Verification items for the finished model (mm, model axes). A direction names the side the tool comes from. Give positions to 0.01 mm unless a question says otherwise; leave off trailing zeros. Write each loop counter-clockwise with the first axis right and the second up, starting at its lowest first coordinate (ties: lowest second). Pieces come first, ordered by that corner, then holes. Notation, with made-up numbers: (-1, -10) -> (14, -10) arc R24 cw to (14, 0) -> close; hole circle Ø4 at (17, -29). An arc over 180 degrees is marked (long way). Use CSV: the item, a comma, the result in double quotes. Start each with the question number.
```python
from build123d import *

# Parameters (mm, degrees)
SKETCH1_W           = 17.5
SKETCH1_H           = 7.5
BOSS_EXTRUDE1_DEPTH = 8.5
SKETCH2_W           = 5.5
SKETCH2_H           = 3.8
BOSS_EXTRUDE2_DEPTH = 5
FILLET1_R           = 1
FILLET2_R           = 1


with BuildPart() as part:
    # Sketch1 → Boss-Extrude1 (new body)
    with BuildSketch(Plane.XY):
        Rectangle(SKETCH1_W, SKETCH1_H)
    extrude(amount=BOSS_EXTRUDE1_DEPTH)

    # Sketch2 → Boss-Extrude2 (add)
    with BuildSketch(Plane.XY.offset(8.5)):
        with Locations((1.6, 0)):
            Rectangle(SKETCH2_W, SKETCH2_H)
    extrude(amount=BOSS_EXTRUDE2_DEPTH)

    # Fillet1
    fillet1_edges = [part.edges().sort_by_distance(p)[0] for p in [
        (8.75, -3.75, 4.25),
        (-8.75, -3.75, 4.25),
        (-8.75, 3.75, 4.25),
        (8.75, 3.75, 4.25),
    ]]
    fillet(fillet1_edges, radius=FILLET1_R)

    # Fillet2
    fillet2_edges = [part.edges().sort_by_distance(p)[0] for p in [
        (8.75, 0, 8.5),
        (0, -3.75, 8.5),
        (0, 3.75, 8.5),
        (-8.75, 0, 8.5),
        (-8.457106781, 3.457106781, 8.5),
        (-8.457106781, -3.457106781, 8.5),
        (8.457106781, 3.457106781, 8.5),
        (8.457106781, -3.457106781, 8.5),
    ]]
    fillet(fillet2_edges, radius=FILLET2_R)


solid = part.part
```
(1) Section check B-B on x = 1. Record the cut outline in (y, z), then the cut area to 3 significant figures.
(2) Section check A-A on y = 0.75. Record the cut outline in (x, z).
(3) Go/stop test with flat-tipped pins: pin 1 (1.1 mm diameter, centred on y = 0, z = 11.5, fed in from +X); pin 2 (8 mm diameter, centred on x = 3, z = 12, fed in from -Y); pin 3 (5.5 mm diameter, centred on x = 2.5, z = 11.5, fed in from -Y). Record where each tip stops, or that it passes through.
(4) Section check D-D on x = 7. Record the cut outline in (y, z).
(5) Thickness scan on line 1 (Z direction, x = -6, y = 0.75); line 2 (X direction, y = 0, z = 10); line 3 (Y direction, x = 3.5, z = 13.25). Record the ranges inside material, lowest first. Write a range as from..to.
(6) Set-up check for faces 1 (the face through (4.35, 0, 11)), 2 (the face through (-1.15, 0, 11)), 3 (the face through (2, 1.9, 11)), 4 (the face through (2, -1.9, 11)): record each of +Z, -Z, +X, -X, +Y, -Y from which the full face is reachable in a straight line by a thin tool's end or side.
(7) Section check C-C on z = 12. Record the cut outline in (x, y), then the cut area to 3 significant figures.
Data:
1,outline,"(-3.75, 0) -> (3.75, 0) -> (3.75, 7.5) arc R1 ccw to (2.75, 8.5) -> (1.9, 8.5) -> (1.9, 13.5) -> (-1.9, 13.5) -> (-1.9, 8.5) -> (-2.75, 8.5) arc R1 ccw to (-3.75, 7.5) -> close"
1,area,"82.3 mm2"
2,outline,"(-8.75, 0) -> (8.75, 0) -> (8.75, 7.5) arc R1 ccw to (7.75, 8.5) -> (4.35, 8.5) -> (4.35, 13.5) -> (-1.15, 13.5) -> (-1.15, 8.5) -> (-7.75, 8.5) arc R1 ccw to (-8.75, 7.5) -> close"
3,pin 1,"stops at x = 4.35"
3,pin 2,"stops at y = -3.62"
3,pin 3,"stops at y = -1.9"
4,outline,"(-3.75, 0) -> (3.75, 0) -> (3.75, 7.5) arc R1 ccw to (2.75, 8.5) -> (-2.75, 8.5) arc R1 ccw to (-3.75, 7.5) -> close"
5,line 1,"z = 0..8.5"
5,line 2,"x = -1.15..4.35"
5,line 3,"y = -1.9..1.9"
6,face 1,"+Z, +X, +Y, -Y"
6,face 2,"+Z, -X, +Y, -Y"
6,face 3,"+Z, +X, -X, +Y"
6,face 4,"+Z, +X, -X, -Y"
7,outline,"(-1.15, -1.9) -> (4.35, -1.9) -> (4.35, 1.9) -> (-1.15, 1.9) -> close"
7,area,"20.9 mm2"
